Drawing for the job (mm, zero at the part's lowest x, y, z). A direction names the side the tool comes from. Give positions to 0.01 mm unless a question says otherwise; leave off trailing zeros. Order: outer loops, then holes, each group sorted by start corner. A loop starts at its lowest first (then second) coordinate and runs counter-clockwise, first axis right, second up. Notation, with made-up numbers: (23.5, 69) - (50.5, 69) arc R14 ccw to (50.5, 86) - close; hole circle Ø1 at (74.25, 73.5). An arc over 180 degrees is marked (long way). One line per item, written item: value.
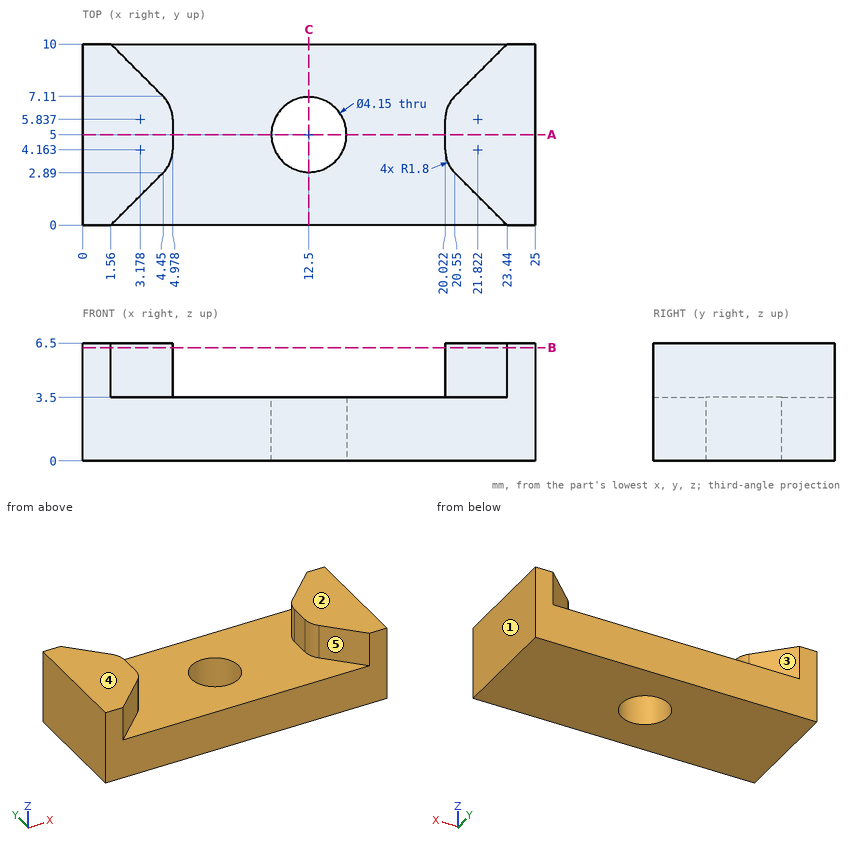
(1) Drill centre lines: line 1 (Y direction, x = 12.5, z = 1.8) (1 decimal); line 2 (Z direction, x = 17.5, y = 8); line 3 (X direction, y = 4.5, z = 5.25). Where is each one in solid material? Low to high.
Completed:
line 1: 0 to 2.9, 7.1 to 10
line 2: 0 to 3.5
line 3: 0 to 4.98, 20.02 to 25
(2) Slice it at A-A, the plane y = 5. Give the cut face in (x, z) (1 decimal).
Completed:
outline: (0, 0) - (10.4, 0) - (10.4, 3.5) - (5, 3.5) - (5, 6.5) - (0, 6.5) - close; (14.6, 0) - (25, 0) - (25, 6.5) - (20, 6.5) - (20, 3.5) - (14.6, 3.5) - close
(3) Slice it at B-B, the plane z = 6.25. Give the cut face in (x, y).
Completed:
outline: (0, 0) - (1.56, 0) - (4.45, 2.89) arc R1.8 ccw to (4.98, 4.16) - (4.98, 5.84) arc R1.8 ccw to (4.45, 7.11) - (1.56, 10) - (0, 10) - close; (20.02, 4.16) arc R1.8 ccw to (20.55, 2.89) - (23.44, 0) - (25, 0) - (25, 10) - (23.44, 10) - (20.55, 7.11) arc R1.8 ccw to (20.02, 5.84) - close
(4) Pin check, flat tips, straight feed: P1, Ø2, axis at x = 6, z = 3, coming from the -Y side; P2, Ø5, axis at x = 12.5, y = 6, coming from the +Z side. Stop position of each tip, or through.
Completed:
P1: y = 0
P2: z = 3.5
(5) 3-axis set-ups, long thin cutter, end or side, ignore diameter. For the marked faces 4 and 5: which of +Z, -Z, +X, -X, +Y, -Y reach the whole face in a straight line?
Completed:
face 4: +Z, +X, -X, +Y, -Y
face 5: +Z, -Y
(6) Slice it at C-C, the plane x = 12.5. Give the cut face in (y, z) (1 decimal).
Completed:
outline: (0, 0) - (2.9, 0) - (2.9, 3.5) - (0, 3.5) - close; (7.1, 0) - (10, 0) - (10, 3.5) - (7.1, 3.5) - close
(7) Pull direction X, two halves, no side cores. Call the marked faces 1, 2 and 3: +X half, -X half, draft (parallel to the pull), parting line (faces both ways), or undercut.
Completed:
face 1: +X half
face 2: draft
face 3: undercut
